Verification items for the finished model (mm, model axes). A direction names the side the tool comes from. Coordinates: 2 decimals unless noted, no trailing zeros. Answer as CSV lines item,"result". Start each with the question number.
1. Set-up check for faces 1 (the flat face through (11, 20, 246)), 2 (the flat face through (0, -7.75, 246)): record each of +Z, -Z, +X, -X, +Y, -Y from which the full face is reachable in a straight line by a thin tool's end or side.
2. Material ranges on L1, parallel to Y at x = -13, z = 34; L2, parallel to Y at x = 0, z = 145, recorded low to high. Write a range as [from, to].
3. Mould release check, pull along X, two halves, no side actions. Record for faces 3 (the flat face through (11, -20, 246)), 4 (the flat face through (-20, 11, 246)), 5 (the flat face through (-7.75, 0, 246)): pulls with the +X half, pulls with the -X half, needs draft (parallel to the pull), parting line crosses it, or undercut.
4. Go/stop test with flat-tipped pins: pin 1 (8.5 mm diameter, centred on y = 1, z = 197, fed in from +X); pin 2 (0.6 mm diameter, centred on x = -17.5, z = 293, fed in from +Y); pin 3 (6 mm diameter, centred on x = -6.5, y = -9.5, fed in from -Z); pin 4 (3.5 mm diameter, centred on x = 0, z = 223, fed in from +Y). Record where each tip stops, or that it passes through.
5. Section check A-A (z = 206). Count the separate pieces of the cut face and the enclosed holes in it, and give its area (3 significant figures).
from build123d import *

# Parameters (mm, degrees)
SKETCH1_R           = 3.35
BOSS_EXTRUDE1_DEPTH = 500


with BuildPart() as part:
    # Sketch1 → Boss-Extrude1 (new body)
    with BuildSketch(Plane.XY):
        with BuildLine():
            Line((-9.853553391, -11.978553391), (-5.771446609, -7.896446609))
            ThreePointArc((-5.771446609, -7.896446609), (-5.609234935, -7.788060234), (-5.417893219, -7.75))
            Line((-5.417893219, -7.75), (5.417893219, -7.75))
            ThreePointArc((5.417893219, -7.75), (5.609234935, -7.788060234), (5.771446609, -7.896446609))
            Line((5.771446609, -7.896446609), (9.853553391, -11.978553391))
            ThreePointArc((9.853553391, -11.978553391), (9.961939766, -12.140765065), (10, -12.332106781))
            Line((10, -12.332106781), (10, -16))
            ThreePointArc((10, -16), (9.707106781, -16.707106781), (9, -17))
            Line((9, -17), (8, -17))
            ThreePointArc((8, -17), (7.292893219, -16.707106781), (7, -16))
            ThreePointArc((7, -16), (6.853553391, -15.646446609), (6.5, -15.5))
            Line((6.5, -15.5), (5, -15.5))
            ThreePointArc((5, -15.5), (4.292893219, -15.792893219), (4, -16.5))
            Line((4, -16.5), (4, -18.5))
            ThreePointArc((4, -18.5), (4.439339828, -19.560660172), (5.5, -20))
            Line((5.5, -20), (17, -20))
            ThreePointArc((17, -20), (19.121320344, -19.121320344), (20, -17))
            Line((20, -17), (20, -5.5))
            ThreePointArc((20, -5.5), (19.560660172, -4.439339828), (18.5, -4))
            Line((18.5, -4), (16.5, -4))
            ThreePointArc((16.5, -4), (15.792893219, -4.292893219), (15.5, -5))
            Line((15.5, -5), (15.5, -6.5))
            ThreePointArc((15.5, -6.5), (15.646446609, -6.853553391), (16, -7))
            ThreePointArc((16, -7), (16.707106781, -7.292893219), (17, -8))
            Line((17, -8), (17, -9))
            ThreePointArc((17, -9), (16.707106781, -9.707106781), (16, -10))
            Line((16, -10), (12.332106781, -10))
            ThreePointArc((12.332106781, -10), (12.140765065, -9.961939766), (11.978553391, -9.853553391))
            Line((11.978553391, -9.853553391), (7.896446609, -5.771446609))
            ThreePointArc((7.896446609, -5.771446609), (7.788060234, -5.609234935), (7.75, -5.417893219))
            Line((7.75, -5.417893219), (7.75, 5.417893219))
            ThreePointArc((7.75, 5.417893219), (7.788060234, 5.609234935), (7.896446609, 5.771446609))
            Line((7.896446609, 5.771446609), (11.978553391, 9.853553391))
            ThreePointArc((11.978553391, 9.853553391), (12.140765065, 9.961939766), (12.332106781, 10))
            Line((12.332106781, 10), (16, 10))
            ThreePointArc((16, 10), (16.707106781, 9.707106781), (17, 9))
            Line((17, 9), (17, 8))
            ThreePointArc((17, 8), (16.707106781, 7.292893219), (16, 7))
            ThreePointArc((16, 7), (15.646446609, 6.853553391), (15.5, 6.5))
            Line((15.5, 6.5), (15.5, 5))
            ThreePointArc((15.5, 5), (15.792893219, 4.292893219), (16.5, 4))
            Line((16.5, 4), (18.5, 4))
            ThreePointArc((18.5, 4), (19.560660172, 4.439339828), (20, 5.5))
            Line((20, 5.5), (20, 17))
            ThreePointArc((20, 17), (19.121320344, 19.121320344), (17, 20))
            Line((17, 20), (5.5, 20))
            ThreePointArc((5.5, 20), (4.439339828, 19.560660172), (4, 18.5))
            Line((4, 18.5), (4, 16.5))
            ThreePointArc((4, 16.5), (4.292893219, 15.792893219), (5, 15.5))
            Line((5, 15.5), (6.5, 15.5))
            ThreePointArc((6.5, 15.5), (6.853553391, 15.646446609), (7, 16))
            ThreePointArc((7, 16), (7.292893219, 16.707106781), (8, 17))
            Line((8, 17), (9, 17))
            ThreePointArc((9, 17), (9.707106781, 16.707106781), (10, 16))
            Line((10, 16), (10, 12.332106781))
            ThreePointArc((10, 12.332106781), (9.961939766, 12.140765065), (9.853553391, 11.978553391))
            Line((9.853553391, 11.978553391), (5.771446609, 7.896446609))
            ThreePointArc((5.771446609, 7.896446609), (5.609234935, 7.788060234), (5.417893219, 7.75))
            Line((5.417893219, 7.75), (-5.417893219, 7.75))
            ThreePointArc((-5.417893219, 7.75), (-5.609234935, 7.788060234), (-5.771446609, 7.896446609))
            Line((-5.771446609, 7.896446609), (-9.853553391, 11.978553391))
            ThreePointArc((-9.853553391, 11.978553391), (-9.961939766, 12.140765065), (-10, 12.332106781))
            Line((-10, 12.332106781), (-10, 16))
            ThreePointArc((-10, 16), (-9.707106781, 16.707106781), (-9, 17))
            Line((-9, 17), (-8, 17))
            ThreePointArc((-8, 17), (-7.292893219, 16.707106781), (-7, 16))
            ThreePointArc((-7, 16), (-6.853553391, 15.646446609), (-6.5, 15.5))
            Line((-6.5, 15.5), (-5, 15.5))
            ThreePointArc((-5, 15.5), (-4.292893219, 15.792893219), (-4, 16.5))
            Line((-4, 16.5), (-4, 18.5))
            ThreePointArc((-4, 18.5), (-4.439339828, 19.560660172), (-5.5, 20))
            Line((-5.5, 20), (-17, 20))
            ThreePointArc((-17, 20), (-19.121320344, 19.121320344), (-20, 17))
            Line((-20, 17), (-20, 5.5))
            ThreePointArc((-20, 5.5), (-19.560660172, 4.439339828), (-18.5, 4))
            Line((-18.5, 4), (-16.5, 4))
            ThreePointArc((-16.5, 4), (-15.792893219, 4.292893219), (-15.5, 5))
            Line((-15.5, 5), (-15.5, 6.5))
            ThreePointArc((-15.5, 6.5), (-15.646446609, 6.853553391), (-16, 7))
            ThreePointArc((-16, 7), (-16.707106781, 7.292893219), (-17, 8))
            Line((-17, 8), (-17, 9))
            ThreePointArc((-17, 9), (-16.707106781, 9.707106781), (-16, 10))
            Line((-16, 10), (-12.332106781, 10))
            ThreePointArc((-12.332106781, 10), (-12.140765065, 9.961939766), (-11.978553391, 9.853553391))
            Line((-11.978553391, 9.853553391), (-7.896446609, 5.771446609))
            ThreePointArc((-7.896446609, 5.771446609), (-7.788060234, 5.609234935), (-7.75, 5.417893219))
            Line((-7.75, 5.417893219), (-7.75, -5.417893219))
            ThreePointArc((-7.75, -5.417893219), (-7.788060234, -5.609234935), (-7.896446609, -5.771446609))
            Line((-7.896446609, -5.771446609), (-11.978553391, -9.853553391))
            ThreePointArc((-11.978553391, -9.853553391), (-12.140765065, -9.961939766), (-12.332106781, -10))
            Line((-12.332106781, -10), (-16, -10))
            ThreePointArc((-16, -10), (-16.707106781, -9.707106781), (-17, -9))
            Line((-17, -9), (-17, -8))
            ThreePointArc((-17, -8), (-16.707106781, -7.292893219), (-16, -7))
            ThreePointArc((-16, -7), (-15.646446609, -6.853553391), (-15.5, -6.5))
            Line((-15.5, -6.5), (-15.5, -5))
            ThreePointArc((-15.5, -5), (-15.792893219, -4.292893219), (-16.5, -4))
            Line((-16.5, -4), (-18.5, -4))
            ThreePointArc((-18.5, -4), (-19.560660172, -4.439339828), (-20, -5.5))
            Line((-20, -5.5), (-20, -17))
            ThreePointArc((-20, -17), (-19.121320344, -19.121320344), (-17, -20))
            Line((-17, -20), (-5.5, -20))
            ThreePointArc((-5.5, -20), (-4.439339828, -19.560660172), (-4, -18.5))
            Line((-4, -18.5), (-4, -16.5))
            ThreePointArc((-4, -16.5), (-4.292893219, -15.792893219), (-5, -15.5))
            Line((-5, -15.5), (-6.5, -15.5))
            ThreePointArc((-6.5, -15.5), (-6.853553391, -15.646446609), (-7, -16))
            ThreePointArc((-7, -16), (-7.292893219, -16.707106781), (-8, -17))
            Line((-8, -17), (-9, -17))
            ThreePointArc((-9, -17), (-9.707106781, -16.707106781), (-10, -16))
            Line((-10, -16), (-10, -12.332106781))
            ThreePointArc((-10, -12.332106781), (-9.961939766, -12.140765065), (-9.853553391, -11.978553391))
        make_face()
        Circle(SKETCH1_R, mode=Mode.SUBTRACT)
        with BuildLine():
            Line((-17, 11.78), (-13, 11.78))
            ThreePointArc((-13, 11.78), (-12.137329727, 12.137329727), (-11.78, 13))
            Line((-11.78, 13), (-11.78, 17))
            ThreePointArc((-11.78, 17), (-12.137329727, 17.862670273), (-13, 18.22))
            Line((-13, 18.22), (-17, 18.22))
            ThreePointArc((-17, 18.22), (-17.862670273, 17.862670273), (-18.22, 17))
            Line((-18.22, 17), (-18.22, 13))
            ThreePointArc((-18.22, 13), (-17.862670273, 12.137329727), (-17, 11.78))
        make_face(mode=Mode.SUBTRACT)
        with BuildLine():
            Line((-18.22, -13), (-18.22, -17))
            ThreePointArc((-18.22, -17), (-17.862670273, -17.862670273), (-17, -18.22))
            Line((-17, -18.22), (-13, -18.22))
            ThreePointArc((-13, -18.22), (-12.137329727, -17.862670273), (-11.78, -17))
            Line((-11.78, -17), (-11.78, -13))
            ThreePointArc((-11.78, -13), (-12.137329727, -12.137329727), (-13, -11.78))
            Line((-13, -11.78), (-17, -11.78))
            ThreePointArc((-17, -11.78), (-17.862670273, -12.137329727), (-18.22, -13))
        make_face(mode=Mode.SUBTRACT)
        with BuildLine():
            Line((13, -18.22), (17, -18.22))
            ThreePointArc((17, -18.22), (17.862670273, -17.862670273), (18.22, -17))
            Line((18.22, -17), (18.22, -13))
            ThreePointArc((18.22, -13), (17.862670273, -12.137329727), (17, -11.78))
            Line((17, -11.78), (13, -11.78))
            ThreePointArc((13, -11.78), (12.137329727, -12.137329727), (11.78, -13))
            Line((11.78, -13), (11.78, -17))
            ThreePointArc((11.78, -17), (12.137329727, -17.862670273), (13, -18.22))
        make_face(mode=Mode.SUBTRACT)
        with BuildLine():
            Line((18.22, 13), (18.22, 17))
            ThreePointArc((18.22, 17), (17.862670273, 17.862670273), (17, 18.22))
            Line((17, 18.22), (13, 18.22))
            ThreePointArc((13, 18.22), (12.137329727, 17.862670273), (11.78, 17))
            Line((11.78, 17), (11.78, 13))
            ThreePointArc((11.78, 13), (12.137329727, 12.137329727), (13, 11.78))
            Line((13, 11.78), (17, 11.78))
            ThreePointArc((17, 11.78), (17.862670273, 12.137329727), (18.22, 13))
        make_face(mode=Mode.SUBTRACT)
    extrude(amount=BOSS_EXTRUDE1_DEPTH)


solid = part.part
Evaluation:
1,face 1,"+Z, -Z, +X, -X, +Y"
1,face 2,"+Z, -Z"
2,L1,"y = [-20, -18.22], [-11.78, -10], [10, 11.78], [18.22, 20]"
2,L2,"y = [-7.75, -3.35], [3.35, 7.75]"
3,face 3,"needs draft"
3,face 4,"pulls with the -X half"
3,face 5,"undercut"
4,pin 1,"stops at x = 19.98"
4,pin 2,"stops at y = 19.99"
4,pin 3,"stops at z = 0"
4,pin 4,"stops at y = 7.75"
5,separate pieces,"1"
5,enclosed holes,"5"
5,area,"670 mm²"
